Here's the drawing with two shaded views (mm, measured from the low corner). I have some questions. Coordinates: 2 decimals unless noted, no trailing zeros.
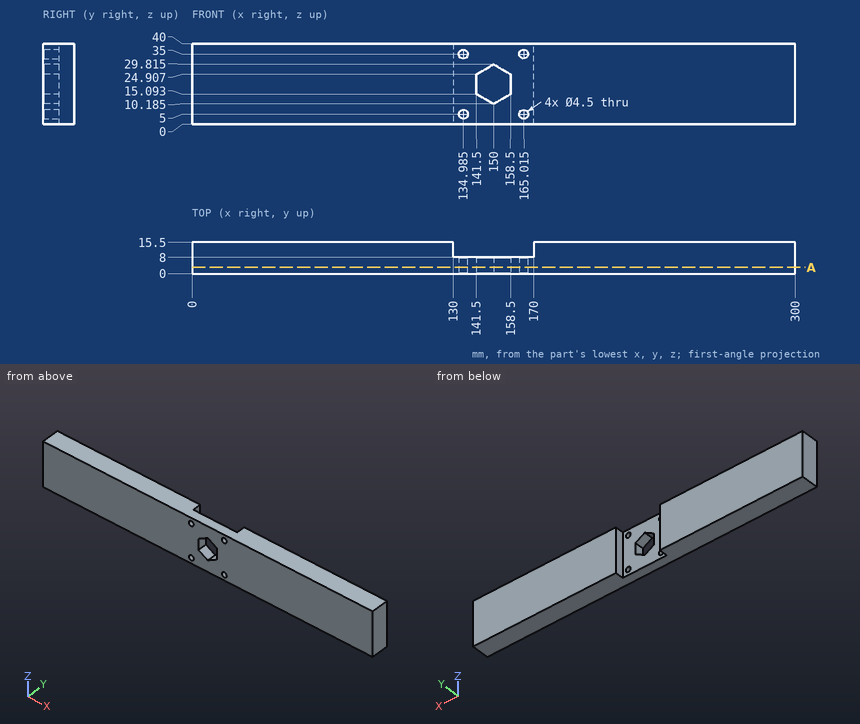
(1) I want a section at A-A on y = 3. State how many separate pieces and enclosed holes the cut face has, then the cut area to 3 significant figures.
Check values:
separate pieces: 1
enclosed holes: 5
area: 11,700 mm2
(2) I'm going to push flat-ended pins straight in: pin 1 (6 mm diameter, centred on y = 5, z = 36, fed in from -X); pin 2 (12 mm diameter, centred on x = 140.5, z = 23, fed in from +Y); pin 3 (4 mm diameter, centred on x = 165.015, z = 5, fed in from -Y). Where does each tip first touch, or does it pass through?
Check values:
pin 1: stops at x = 0
pin 2: stops at y = 8
pin 3: passes through
(3) If I drill on probe 1 along X at (y, z) = (14.25, 4); probe 2 along Y at (x, z) = (151.5, 34); probe 3 along X at (y, z) = (3, 11.5) (1 decimal), over which ranges is the centre line in solid material (lowest first)?
Check values:
probe 1: x = 0 to 130, 170 to 300
probe 2: y = 0 to 8
probe 3: x = 0 to 147.7, 152.3 to 300
